Here's how the part is built. I have some questions about the finished solid (model axes, mm). Face numbers are marked on the shaded views. A direction names the side the tool comes from. Round coordinates to 2 decimals unless told otherwise and drop trailing zeros. Loops run counter-clockwise (first coordinate to the right, second up) from the corner with the lowest first, then second, coordinate; pieces in that order, holes last. Notation, with made-up numbers: M 62.25,35.25 L 112.25,35.25 A15 cw 112.25,52.25 Z; hole C 3.5,-12 d10. An arc over 180 degrees is marked long. Use a Markdown table: item, result.
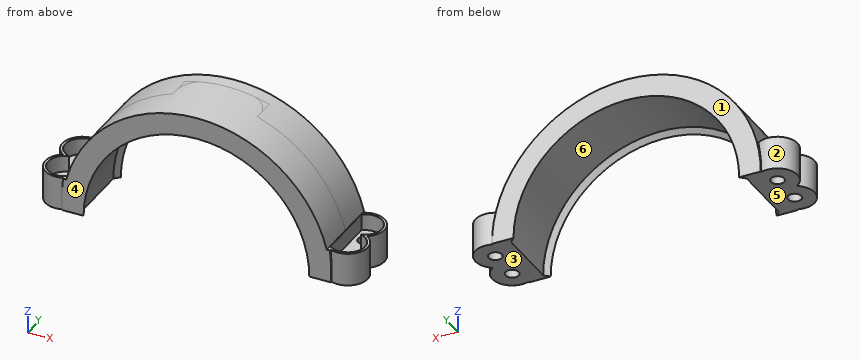
from build123d import *

# Parameters (mm, degrees)
REVOLVE1_ANGLE                  = 180
BOSS_EXTRUDE1_START             = -11
BOSS_EXTRUDE1_DEPTH             = 11
CUT_EXTRUDE1_REACH              = 68.374
BOSS_EXTRUDE2_REACH             = 67.327
BOSS_EXTRUDE2_END_RADIUS        = 40.5
SKETCH6_W                       = 25.4
SKETCH6_H                       = 18
BOSS_EXTRUDE2_DIRECTION_2_DEPTH = 15
SKETCH8_W                       = 4
SKETCH8_H                       = 19.884534
CUT_EXTRUDE3_DEPTH              = 80.722348
FILLET1_START                   = 2
FILLET1_DEPTH                   = 5
FILLET1_START_2                 = -11
FILLET1_2_DEPTH                 = 16.09884
FILLET1_START_3                 = 37
FILLET1_3_DEPTH                 = 28
FILLET1_START_4                 = 62
FILLET1_4_OUTLINE_W             = 4
FILLET1_4_OUTLINE_H             = 5
FILLET1_4_DEPTH                 = 3
FILLET1_START_5                 = 39.17071
FILLET1_5_OUTLINE_W             = 4
FILLET1_5_OUTLINE_H             = 5
FILLET1_5_DEPTH                 = 2.944756
FILLET1_6_DEPTH                 = 6
SKETCH9_R                       = 2
BOSS_EXTRUDE3_DEPTH             = 10
CUT_EXTRUDE4_DEPTH              = 75.187772
CUT_EXTRUDE4_DEPTH_BACK         = 5
CUT_EXTRUDE5_DEPTH              = 85.064413


with BuildPart() as part:
    # Sketch2 → Revolve1 (revolve, symmetric)
    with BuildSketch(Plane(origin=(0, 0, 0), x_dir=(0, 0, -1), z_dir=(1, 0, 0))) as revolve1_sk:
        Polygon((-34, -11), (-35.5, -9.5), (-35.5, 9.5), (-34, 11), (-35.5, 11), (-40.5, 11), (-40.5, -11), (-35.5, -11), align=None)
    revolve(axis=Axis((0, 0, 0), (0, 1, 0)), revolution_arc=REVOLVE1_ANGLE / 2)
    revolve(revolve1_sk.sketch, axis=Axis((0, 0, 0), (0, -1, 0)), revolution_arc=REVOLVE1_ANGLE / 2)

    # Sketch3 → Boss-Extrude1 (add)
    with BuildSketch(Plane(origin=(0, 0, 0), x_dir=(1, 0, 0), z_dir=(0, 1, 0)).offset(BOSS_EXTRUDE1_START)):
        with BuildLine():
            ThreePointArc((-40.5, 0), (0, -40.5), (40.5, 0))
            add(Edge.make_bspline(
                [(40.5, 0), (41.574904, -20.679763), (31.861074, -51.110818), (0, -51.360442)],
                knots=[0, 0, 0, 0, 1, 1, 1, 1], degree=3))
            add(Edge.make_bspline(
                [(-40.5, 0), (-41.574904, -20.679763), (-31.861074, -51.110818), (0, -51.360442)],
                knots=[0, 0, 0, 0, 1, 1, 1, 1], degree=3))
        make_face()
    extrude(amount=BOSS_EXTRUDE1_DEPTH)

    # Sketch5 → Cut-Extrude1 (cut, up to next)
    with BuildSketch(Plane(origin=(0, 0, 0), x_dir=(1, 0, 0), z_dir=(0, 1, 0)), mode=Mode.PRIVATE) as cut_extrude1_sk1:
        Polygon((32.298595, -50), (-32.298595, -50), (-4.520904, -70.798059), align=None)
    cut_extrude1_tool1 = extrude(cut_extrude1_sk1.sketch, amount=-CUT_EXTRUDE1_REACH, mode=Mode.PRIVATE) & part.part
    add(cut_extrude1_tool1.solids().sort_by_distance((-1.506968, 0, 56.932686))[0], mode=Mode.SUBTRACT)

    # Boss-Extrude2: up to this cylinder (the profile starts outside it)
    boss_extrude2_end = Plane(origin=(0, -2, 0), z_dir=(0, -1, 0)) * Cylinder(BOSS_EXTRUDE2_END_RADIUS, 216.654, mode=Mode.PRIVATE)
    # Sketch6 → Boss-Extrude2 (add, up to the surface)
    with BuildSketch(Plane.XY.offset(50), mode=Mode.PRIVATE) as boss_extrude2_sk1:
        with Locations((0, -2)):
            Rectangle(SKETCH6_W, SKETCH6_H)
    boss_extrude2_tool1 = extrude(boss_extrude2_sk1.sketch, amount=-BOSS_EXTRUDE2_REACH, mode=Mode.PRIVATE) - boss_extrude2_end
    add(boss_extrude2_tool1.solids().sort_by_distance((0, -2, 50))[0])

    # Sketch6 → Boss-Extrude2 direction 2 (add)
    with BuildSketch(Plane.XY.offset(50)):
        with Locations((0, -2)):
            Rectangle(SKETCH6_W, SKETCH6_H)
    extrude(amount=BOSS_EXTRUDE2_DIRECTION_2_DEPTH)

    # Sketch8 → Cut-Extrude3 (cut, through all)
    with BuildSketch(Plane(origin=(0, 11, 0), x_dir=(1, 0, 0), z_dir=(0, 1, 0))):
        with BuildLine():
            Line((15.113165, -40.129156), (15.113165, -45.006528))
            add(Edge.make_bspline(
                [(15.113165, -45.006528), (20.553217, -43.096096), (30.745136, -32.716473), (33.442003, -26.840069)],
                knots=[0, 0, 0, 0, 1, 1, 1, 1], degree=3))
            ThreePointArc((33.442003, -26.840069), (25.17044, -34.716075), (15.113165, -40.129156))
        make_face()
        with BuildLine():
            Line((-15.113165, -40.129156), (-15.113165, -45.006528))
            add(Edge.make_bspline(
                [(-15.113165, -45.006528), (-20.553217, -43.096096), (-30.745136, -32.716473), (-33.442003, -26.840069)],
                knots=[0, 0, 0, 0, 1, 1, 1, 1], degree=3))
            ThreePointArc((-33.442003, -26.840069), (-25.17044, -34.716075), (-15.113165, -40.129156))
        make_face()
        with Locations((0, -52.057733)):
            Rectangle(SKETCH8_W, SKETCH8_H)
    extrude(amount=-CUT_EXTRUDE3_DEPTH, mode=Mode.SUBTRACT)

    # Fillet1: read off the stored shape, not the designer's step
    # Fillet1 outline → Fillet1 (cut)
    with BuildSketch(Plane(origin=(0, 0, 0), x_dir=(1, 0, 0), z_dir=(0, 1, 0)).offset(FILLET1_START)):
        with BuildLine():
            Line((-12.7, -65), (12.7, -65))
            Line((12.7, -65), (12.7, -38.457249))
            ThreePointArc((12.7, -38.457249), (0, -40.5), (-12.7, -38.457249))
            Line((-12.7, -38.457249), (-12.7, -65))
        make_face()
    extrude(amount=FILLET1_DEPTH, mode=Mode.SUBTRACT)

    # Fillet1 2 outline → Fillet1 2 (cut)
    with BuildSketch(Plane(origin=(0, 0, 0), x_dir=(1, 0, 0), z_dir=(0, 1, 0)).offset(FILLET1_START_2)):
        with BuildLine():
            Line((-12.7, -65), (-7.7, -65))
            add(Edge.make_bspline(
                [(-7.7, -65), (-12.7, -65), (-12.7, -60)],
                knots=[0, 0, 0, 1, 1, 1], degree=2, weights=[1, 0.707107, 1]))
            Line((-12.7, -60), (-12.7, -65))
        make_face()
        with BuildLine():
            add(Edge.make_bspline(
                [(7.7, -65), (12.7, -65), (12.7, -60)],
                knots=[0, 0, 0, 1, 1, 1], degree=2, weights=[1, 0.707107, 1]))
            Line((7.7, -65), (12.7, -65))
            Line((12.7, -65), (12.7, -60))
        make_face()
    extrude(amount=FILLET1_2_DEPTH, mode=Mode.SUBTRACT)

    # Fillet1 3 outline → Fillet1 3 (add)
    with BuildSketch(Plane.XY.offset(FILLET1_START_3)):
        with BuildLine():
            add(Edge.make_bspline(
                [(-12.7, 2), (-12.7, 7), (-7.7, 7)],
                knots=[0, 0, 0, 1, 1, 1], degree=2, weights=[1, 0.707107, 1]))
            Line((-12.7, 2), (-2, 2))
            Line((-2, 2), (-2, 7))
            Line((-2, 7), (-7.7, 7))
        make_face()
        with BuildLine():
            Line((2, 7), (2, 2))
            Line((2, 2), (12.7, 2))
            add(Edge.make_bspline(
                [(7.7, 7), (12.7, 7), (12.7, 2)],
                knots=[0, 0, 0, 1, 1, 1], degree=2, weights=[1, 0.707107, 1]))
            Line((7.7, 7), (2, 7))
        make_face()
    extrude(amount=FILLET1_3_DEPTH)

    # Fillet1 4 outline → Fillet1 4 (add)
    with BuildSketch(Plane.XY.offset(FILLET1_START_4)):
        with Locations((0, 4.5)):
            Rectangle(FILLET1_4_OUTLINE_W, FILLET1_4_OUTLINE_H)
    extrude(amount=FILLET1_4_DEPTH)

    # Fillet1 5 outline → Fillet1 5 (add)
    with BuildSketch(Plane.XY.offset(FILLET1_START_5)):
        with Locations((0, 4.5)):
            Rectangle(FILLET1_5_OUTLINE_W, FILLET1_5_OUTLINE_H)
    extrude(amount=FILLET1_5_DEPTH)

    # Fillet1 6 outline → Fillet1 6 (cut)
    with BuildSketch(Plane(origin=(0, 0, 0), x_dir=(1, 0, 0), z_dir=(0, 1, 0)).offset(FILLET1_START)):
        with BuildLine():
            Line((-12.7, -65), (-7.7, -65))
            add(Edge.make_bspline(
                [(-12.7, -60), (-12.7, -60.274102), (-12.679965, -60.548369), (-12.639842, -60.820553), (-12.536378, -61.284433), (-12.482162, -61.478121), (-12.41762, -61.668662), (-12.288664, -61.991396), (-12.22893, -62.125441), (-12.163988, -62.25706), (-11.922281, -62.702191), (-11.720174, -63.002028), (-11.490067, -63.281001), (-10.981001, -63.790067), (-10.702028, -64.020174), (-10.402191, -64.222281), (-9.95706, -64.463988), (-9.825441, -64.52893), (-9.691396, -64.588664), (-9.368662, -64.71762), (-9.178121, -64.782162), (-8.984433, -64.836378), (-8.520553, -64.939842), (-8.248369, -64.979965), (-7.974102, -65), (-7.7, -65)],
                knots=[0, 0, 0, 0, 0, 0.139857, 0.139857, 0.139857, 0.242164, 0.242164, 0.242164, 0.316823, 0.316823, 0.316823, 0.5, 0.5, 0.5, 0.683177, 0.683177, 0.683177, 0.757836, 0.757836, 0.757836, 0.860143, 0.860143, 0.860143, 1, 1, 1, 1, 1], degree=4))
            Line((-12.7, -60), (-12.7, -65))
        make_face()
        with BuildLine():
            Line((12.7, -65), (12.7, -60))
            add(Edge.make_bspline(
                [(12.7, -60), (12.7, -60.274102), (12.679965, -60.548369), (12.639842, -60.820553), (12.536378, -61.284433), (12.482162, -61.478121), (12.41762, -61.668662), (12.288664, -61.991396), (12.22893, -62.125441), (12.163988, -62.25706), (11.922281, -62.702191), (11.720174, -63.002028), (11.490067, -63.281001), (10.981001, -63.790067), (10.702028, -64.020174), (10.402191, -64.222281), (9.95706, -64.463988), (9.825441, -64.52893), (9.691396, -64.588664), (9.368662, -64.71762), (9.178121, -64.782162), (8.984433, -64.836378), (8.520553, -64.939842), (8.248369, -64.979965), (7.974102, -65), (7.7, -65)],
                knots=[0, 0, 0, 0, 0, 0.139857, 0.139857, 0.139857, 0.242164, 0.242164, 0.242164, 0.316823, 0.316823, 0.316823, 0.5, 0.5, 0.5, 0.683177, 0.683177, 0.683177, 0.757836, 0.757836, 0.757836, 0.860143, 0.860143, 0.860143, 1, 1, 1, 1, 1], degree=4))
            Line((7.7, -65), (12.7, -65))
        make_face()
    extrude(amount=FILLET1_6_DEPTH, mode=Mode.SUBTRACT)

    # Sketch9 → Boss-Extrude3 (add)
    # profile 1 of 2: a face of its own
    with BuildSketch(Plane.XY):
        with BuildLine():
            ThreePointArc((39.222943, -0.011905), (42.578982, -10.999961), (45.856052, 0.011905))
            ThreePointArc((45.856052, 0.011905), (42.500013, 10.999961), (39.222943, -0.011905))
        make_face()
        with Locations((42.557445, -5)):
            Circle(SKETCH9_R, mode=Mode.SUBTRACT)
        with Locations((42.52155, 5)):
            Circle(SKETCH9_R, mode=Mode.SUBTRACT)
    # profile 2 of 2: a face of its own
    with BuildSketch(Plane.XY):
        with BuildLine():
            ThreePointArc((-39.222943, -0.011905), (-42.578982, -10.999961), (-45.856052, 0.011905))
            ThreePointArc((-45.856052, 0.011905), (-42.500013, 10.999961), (-39.222943, -0.011905))
        make_face()
        with Locations(Location((-42.557445, -5, 0), (0, 0, 180))):
            Circle(SKETCH9_R, mode=Mode.SUBTRACT)
        with Locations(Location((-42.52155, 5, 0), (0, 0, 180))):
            Circle(SKETCH9_R, mode=Mode.SUBTRACT)
    extrude(amount=BOSS_EXTRUDE3_DEPTH)

    # Sketch10 → Cut-Extrude4 (cut, two sides: drawn at the far end of the back side and taken through both)
    with BuildSketch(Plane.XY.offset(10).offset(-CUT_EXTRUDE4_DEPTH_BACK)):
        with BuildLine():
            Line((39.407769, -9.137577), (39.407769, 9.164657))
            ThreePointArc((39.407769, 9.164657), (47.176604, 7.317427), (43.967661, 0.005126))
            ThreePointArc((43.967661, 0.005126), (47.210797, -7.320844), (39.407769, -9.137577))
        make_face()
        with BuildLine():
            Line((-39.407769, -9.137577), (-39.407769, 9.164657))
            ThreePointArc((-39.407769, 9.164657), (-47.176604, 7.317427), (-43.967661, 0.005126))
            ThreePointArc((-43.967661, 0.005126), (-47.210797, -7.320844), (-39.407769, -9.137577))
        make_face()
    extrude(amount=CUT_EXTRUDE4_DEPTH + CUT_EXTRUDE4_DEPTH_BACK, mode=Mode.SUBTRACT)

    # Sketch11 → Cut-Extrude5 (cut, through all)
    with BuildSketch(Plane(origin=(0, 11, 0), x_dir=(1, 0, 0), z_dir=(0, 1, 0))):
        with BuildLine():
            Line((48.52155, -10), (39.246019, -10))
            ThreePointArc((39.246019, -10), (0, -40.5), (-39.246019, -10))
            Line((-39.246019, -10), (-48.52155, -10))
            Line((-48.52155, -10), (-48.52155, -69.748878))
            Line((-48.52155, -69.748878), (48.52155, -69.748878))
            Line((48.52155, -69.748878), (48.52155, -10))
        make_face()
    extrude(amount=-CUT_EXTRUDE5_DEPTH, mode=Mode.SUBTRACT)


solid = part.part
1. Imagine slicing it at B-B, the plane x = 0. Write out the boundary of the cut face in (y, z), then the cut area to 3 significant figures.
Answer sheet:
| item | result |
|---|---|
| outline | M -11,34 L -9.5,35.5 L 9.5,35.5 L 11,34 L 11,40.5 L -11,40.5 Z |
| area | 112 mm2 |
2. I need wall thicknesses on probe 1 along X at (y, z) = (4.75, 3); probe 2 along X at (y, z) = (5, 6.45); probe 3 along Z at (x, y) = (39.5, -4.5). Which ranges of each line are inside material? Lowest first, please. Write a range as from..to.
Answer sheet:
| item | result |
|---|---|
| probe 1 | -48.52..-44.51, -40.54..-35.37, 35.37..40.54, 44.51..48.52 |
| probe 2 | -48.52..-47.72, -39.41..-34.91, 34.91..39.41, 47.72..48.52 |
| probe 3 | 0..5 |
3. Which directions (+Z, -Z, +X, -X, +Y, -Y) give clear straight access to the entire face, cutting with the end or side of a thin tool? Please do the marked faces 5 and 6.
Answer sheet:
| item | result |
|---|---|
| face 5 | -Z, +X, -X, +Y, -Y |
| face 6 | -Z |
4. For pin 1 Ø6.5 at (x, y) = (-44, 2) entering from +Z; pin 2 Ø5 at (x, y) = (13.5, 8.5) entering from -Z; pin 3 Ø9 at (x, y) = (42, 1) entering from +Z, each with a flat end and sliding along its axis, tell me the tip position at first contact or that it passes through.
Answer sheet:
| item | result |
|---|---|
| pin 1 | z = 10 |
| pin 2 | z = 30.98 |
| pin 3 | z = 15.3 |
5. We'd pull the mould along Y, two halves only. Please class the marked faces 1, 2, 3 and 4: +Y half, -Y half, draft (parallel to the pull), parting line (faces both ways), or undercut.
Answer sheet:
| item | result |
|---|---|
| face 1 | +Y half |
| face 2 | undercut |
| face 3 | draft |
| face 4 | -Y half |
6. Imagine slicing it at A-A, the plane y = 5. Write out the boundary of the cut face in (x, z), then the cut area to 3 significant figures.
Answer sheet:
| item | result |
|---|---|
| outline | M -48.52,0 L -44.52,0 L -44.52,5 L -47.72,5 L -47.72,10 L -48.52,10 Z; M -40.52,0 L -35.5,0 A35.5 cw 35.5,0 L 40.52,0 L 40.52,5 L 39.41,5 L 39.41,10 L 39.25,10 A40.5 ccw -39.25,10 L -39.41,10 L -39.41,5 L -40.52,5 Z; M 44.52,0 L 48.52,0 L 48.52,10 L 47.72,10 L 47.72,5 L 44.52,5 Z |
| area | 643 mm2 |
